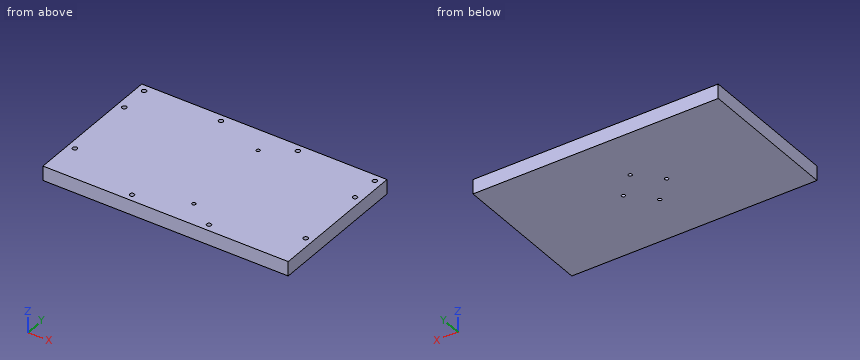
Autodesk Inventor part; units mm, degrees
ref_plane "YZ Plane" through (0, 0, 0) normal (1, 0, 0) x (0, 1, 0)
ref_plane "XZ Plane" through (0, 0, 0) normal (0, 1, 0) x (-1, 0, 0)
ref_plane "XY Plane" through (0, 0, 0) normal (0, 0, 1) x (1, 0, 0)
sketch "Sketch1" plane through (0, 0, 0) normal (0, 0, 1) x (1, 0, 0)
  line L0 (-85, 50) -> (85, 50)
  line L1 (85, 50) -> (85, -50)
  line L2 (85, -50) -> (-85, -50)
  line L3 (-85, -50) -> (-85, 50)
  line L4 (-85, 50) -> (85, -50) construction
  line L5 (85, 50) -> (-85, -50) construction
  point P0 (0, 0)
  dimension "d0" = 170
  dimension "d1" = 100
extrude "Extrusion1" add sketch "Sketch1" along normal mid plane 10
sketch "Sketch2" plane through (0, 0, 5) normal (0, 0, 1) x (1, 0, 0)
  line L0 (-85, 50) -> (-85, -50)
  line L1 (-85, -50) -> (85, -50)
  line L2 (85, -50) -> (85, 50)
  line L3 (85, 50) -> (-85, 50)
  line L4 (-85, 50) -> (-85, -50)
  point P0 (0, 0)
  point P1 (80, 45)
  point P2 (26.6667, 45)
  point P3 (-80, 45)
  point P4 (80, 25)
  point P5 (80, -25)
  point P6 (-80, 25)
  point P7 (-80, -25)
  point P8 (-26.6667, 45)
  point P9 (26.6667, -45)
  point P10 (-26.6667, -45)
  dimension "d17" = 53.3333
  dimension "d53" = 50
  dimension "d61" = 160
  dimension "d68" = 160
  dimension "d73" = 5
  dimension "d74" = 5
  dimension "d75" = 5
  dimension "d77" = 5
  dimension "d112" = 53.3333
  dimension "d115" = 90
  dimension "d118" = 25
hole "Hole1" at (-80, 45, 5) at (26.6667, 45, 5) at (80, 45, 5) at (80, 25, 5) at (80, -25, 5) at (-80, 25, 5) at (-80, -25, 5) at (-26.6667, 45, 5) at (-26.6667, -45, 5) at (26.6667, -45, 5) direction (0, 0, -1) diameter 3.175 depth 5
sketch "Sketch3" plane through (0, 0, -5) normal (0, 0, -1) x (-1, 0, 0)
  point P0 (0, 0)
  point P1 (0, 15)
  point P2 (-15, 0)
  point P3 (0, -15)
  point P4 (15, 0)
  dimension "d81" = 15
  dimension "d84" = 360
hole "Hole2" at (0, 15, -5) at (15, 0, -5) at (0, -15, -5) at (-15, 0, -5) direction (0, 0, 1) diameter 2.5 depth 3
sketch "Sketch4" plane through (0, 0, 5) normal (0, 0, 1) x (1, 0, 0)
  line L0 (85, -50) -> (85, 50)
  line L1 (-85, 50) -> (-85, -50)
  point P0 (0, 0)
  point P1 (7.62, 32.5)
  point P2 (7.62, -32.5)
  dimension "d94" = 32.5
  dimension "d97" = 65
  dimension "d109" = 92.62
hole "Hole3" at (7.62, 32.5, 5) at (7.62, -32.5, 5) direction (0, 0, -1) diameter 2.5 depth 3
properties part number "base"
Could you check a few things on this model? Use its own coordinates, in mm. Coordinates: 2 decimals unless noted, no trailing zeros. Order: outer loops, then holes, each group sorted by start corner. A loop starts at its lowest first (then second) coordinate and runs counter-clockwise, first axis right, second up.
Q1. Will these pins go through, and if not, where does the flat tip stop? pin 1 (2.5 mm diameter, centred on x = -80, y = -25, fed in from +Z); pin 2 (0.8 mm diameter, centred on x = 8, y = 32.5, fed in from +Z).
Q2. Please list where these lines run through material, in increasing order: L1, parallel to X at y = 45, z = 2.8; L2, parallel to X at y = -25, z = 2.7; L3, parallel to Y at x = -80, z = 1.55.
Q3. Suppose I cut it at A-A on x = -80. Please give me the cut outline in (y, z).
Q4. Suppose I cut it at B-B on y = -25. Please give me the cut outline in (x, z), and give its area (3 significant figures).
Answer:
1. pin 1: stops at z = 0
1. pin 2: stops at z = 2
2. L1: x = -85 to -81.59, -78.41 to -28.25, -25.08 to 25.08, 28.25 to 78.41, 81.59 to 85
2. L2: x = -85 to -81.59, -78.41 to 78.41, 81.59 to 85
2. L3: y = -50 to -26.59, -23.41 to 23.41, 26.59 to 43.41, 46.59 to 50
3. outline: (-50, -5) - (50, -5) - (50, 5) - (46.59, 5) - (46.59, 0) - (43.41, 0) - (43.41, 5) - (26.59, 5) - (26.59, 0) - (23.41, 0) - (23.41, 5) - (-23.41, 5) - (-23.41, 0) - (-26.59, 0) - (-26.59, 5) - (-50, 5) - close
4. outline: (-85, -5) - (85, -5) - (85, 5) - (81.59, 5) - (81.59, 0) - (78.41, 0) - (78.41, 5) - (-78.41, 5) - (-78.41, 0) - (-81.59, 0) - (-81.59, 5) - (-85, 5) - close
4. area: 1,670 mm2
